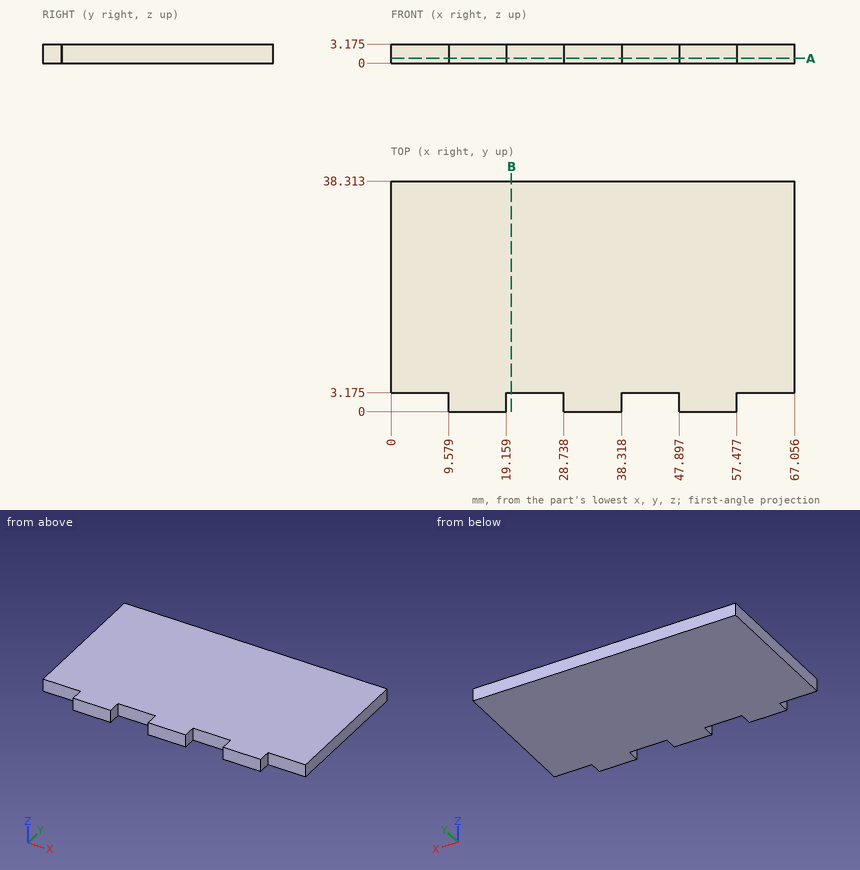
Check sheet for the drawn part. Datum: minimum x, y, z corner. Units: mm. Coordinates: 2 decimals unless noted, no trailing zeros. Order: outer loops, then holes, each group sorted by start corner. A loop starts at its lowest first (then second) coordinate and runs counter-clockwise, first axis right, second up. Notation, with made-up numbers: M 75,80.25 L 102,80.25 A6 cw 102,90.25 Z; hole C 42,87 d2. An arc over 180 degrees is marked long. One line per item, written item: value. Start each with the question number.
Item 1: Gauge pin test, flat ends, axial feed: pin 1 (1.6 mm diameter, centred on x = 44, z = 1, fed in from -Y) (3 decimals); pin 2 (6 mm diameter, centred on x = 23, y = 31, fed in from -Z); pin 3 (1.6 mm diameter, centred on y = 1, z = 2, fed in from +X); pin 4 (1 mm diameter, centred on y = 1.5, z = 2, fed in from -X). Record the tip position at first contact, or that the pin passes through.
Item 2: Sectioned sample at A-A (z = 0.8). Enter the section's corners in (x, y) (1 decimal), then the cut area to 3 significant figures.
Item 3: Sectioned sample at B-B (x = 20). Enter the section's corners in (y, z) (1 decimal).
Item 4: Scan lines: probe 1 along X at (y, z) = (2.5, 2.9); probe 2 along Y at (x, z) = (4, 2.3) (1 decimal). Record each from-to range of solid material in increasing order.
Conclusion:
1. pin 1: stops at y = 3.175
1. pin 2: stops at z = 0
1. pin 3: stops at x = 57.48
1. pin 4: stops at x = 9.58
2. outline: M 0,3.2 L 9.6,3.2 L 9.6,0 L 19.2,0 L 19.2,3.2 L 28.7,3.2 L 28.7,0 L 38.3,0 L 38.3,3.2 L 47.9,3.2 L 47.9,0 L 57.5,0 L 57.5,3.2 L 67.1,3.2 L 67.1,38.3 L 0,38.3 Z
2. area: 2,450 mm^2
3. outline: M 3.2,0 L 38.3,0 L 38.3,3.2 L 3.2,3.2 Z
4. probe 1: x = 9.58 to 19.16, 28.74 to 38.32, 47.9 to 57.48
4. probe 2: y = 3.2 to 38.3
